from build123d import *

# Parameters (mm, degrees)
BASE_FLANGE1_DEPTH      = 2
EDGE_FLANGE1_DEPTH      = 40
EDGE_FLANGE1_BEND_DEPTH = 40
EDGE_FLANGE2_DEPTH      = 40
EDGE_FLANGE2_BEND_DEPTH = 40
SKETCH28_R              = 4
CUT_EXTRUDE1_DEPTH      = 2
SKETCH29_R              = 3
CUT_EXTRUDE2_DEPTH      = 2
SKETCH30_R              = 3
CUT_EXTRUDE3_DEPTH      = 2


# Sheet-metal steps are written as plain solids
with BuildPart() as part:
    # Sketch1 → Base-Flange1 (new body)
    with BuildSketch(Plane.XY):
        Polygon((-225, 173.125), (-225, -173.125), (-185, -173.125), (-185, -98.125), (185, -98.125), (185, -173.125), (225, -173.125), (225, 173.125), (185, 173.125), (185, 143.125), (-185, 143.125), (-185, 173.125), align=None)
    extrude(amount=-BASE_FLANGE1_DEPTH)

    # Edge-Flange1 section (across the edge) → Edge-Flange1 (add)
    with BuildSketch(Plane(origin=(-185, 173.339359354, 0), x_dir=(0, -0.49999999999999495, 0.8660254037844416), z_dir=(-1, 0, 0))):
        with BuildLine():
            Line((-2, 0.214359354), (-2, 38.954101615))
            Line((-2, 38.954101615), (0, 38.954101615))
            Line((0, 38.954101615), (0, 0.214359354))
            ThreePointArc((0, 0.214359354), (0.027259339, 0.007304118), (0.107179677, -0.185640646))
            Line((0.107179677, -0.185640646), (-1.624871131, -1.185640646))
            ThreePointArc((-1.624871131, -1.185640646), (-1.904592314, -0.510333972), (-2, 0.214359354))
        make_face()
    extrude(amount=EDGE_FLANGE1_DEPTH)

    # Edge-Flange1 section 2 (across the edge) → Edge-Flange1 bend (add)
    with BuildSketch(Plane(origin=(225, 173.339359354, 0), x_dir=(0, -0.49999999999999495, 0.8660254037844416), z_dir=(-1, 0, 0))):
        with BuildLine():
            Line((-2, 0.214359354), (-2, 38.954101615))
            Line((-2, 38.954101615), (0, 38.954101615))
            Line((0, 38.954101615), (0, 0.214359354))
            ThreePointArc((0, 0.214359354), (0.027259339, 0.007304118), (0.107179677, -0.185640646))
            Line((0.107179677, -0.185640646), (-1.624871131, -1.185640646))
            ThreePointArc((-1.624871131, -1.185640646), (-1.904592314, -0.510333972), (-2, 0.214359354))
        make_face()
    extrude(amount=EDGE_FLANGE1_BEND_DEPTH)

    # Edge-Flange2 section (across the edge) → Edge-Flange2 (add)
    with BuildSketch(Plane(origin=(-185, -173.339359354, -2), x_dir=(0, 0.49999999999999495, -0.8660254037844416), z_dir=(-1, 0, 0))):
        with BuildLine():
            Line((-2, 0.214359354), (-2, 29.464101615))
            Line((-2, 29.464101615), (0, 29.464101615))
            Line((0, 29.464101615), (0, 0.214359354))
            ThreePointArc((0, 0.214359354), (0.027259339, 0.007304118), (0.107179677, -0.185640646))
            Line((0.107179677, -0.185640646), (-1.624871131, -1.185640646))
            ThreePointArc((-1.624871131, -1.185640646), (-1.904592314, -0.510333972), (-2, 0.214359354))
        make_face()
    extrude(amount=EDGE_FLANGE2_DEPTH)

    # Edge-Flange2 section 2 (across the edge) → Edge-Flange2 bend (add)
    with BuildSketch(Plane(origin=(225, -173.339359354, -2), x_dir=(-1.3877787807814315e-15, 0.49999999999999495, -0.8660254037844416), z_dir=(-1, 0, 0))):
        with BuildLine():
            Line((-2, 0.214359354), (-2, 29.464101615))
            Line((-2, 29.464101615), (0, 29.464101615))
            Line((0, 29.464101615), (0, 0.214359354))
            ThreePointArc((0, 0.214359354), (0.027259339, 0.007304118), (0.107179677, -0.185640646))
            Line((0.107179677, -0.185640646), (-1.624871131, -1.185640646))
            ThreePointArc((-1.624871131, -1.185640646), (-1.904592314, -0.510333972), (-2, 0.214359354))
        make_face()
    extrude(amount=EDGE_FLANGE2_BEND_DEPTH)

    # Sketch28 → Cut-Extrude1 (cut)
    with BuildSketch(Plane.XY):
        with Locations((-205, 143.125)):
            Circle(SKETCH28_R)
        with Locations((-205, 110.125)):
            Circle(SKETCH28_R)
        with Locations((-205, 77.125)):
            Circle(SKETCH28_R)
        with Locations((-205, 44.125)):
            Circle(SKETCH28_R)
        with Locations((-205, 11.125)):
            Circle(SKETCH28_R)
        with Locations((-205, -21.875)):
            Circle(SKETCH28_R)
        with Locations((-205, -54.875)):
            Circle(SKETCH28_R)
        with Locations((-205, -87.875)):
            Circle(SKETCH28_R)
        with Locations((-205, -120.875)):
            Circle(SKETCH28_R)
        with Locations((-205, -153.875)):
            Circle(SKETCH28_R)
        with Locations(Location((205, -153.875, 0), (0, 0, 180))):
            Circle(SKETCH28_R)
        with Locations(Location((205, -120.875, 0), (0, 0, 180))):
            Circle(SKETCH28_R)
        with Locations(Location((205, -87.875, 0), (0, 0, 180))):
            Circle(SKETCH28_R)
        with Locations(Location((205, -54.875, 0), (0, 0, 180))):
            Circle(SKETCH28_R)
        with Locations(Location((205, -21.875, 0), (0, 0, 180))):
            Circle(SKETCH28_R)
        with Locations(Location((205, 11.125, 0), (0, 0, 180))):
            Circle(SKETCH28_R)
        with Locations(Location((205, 44.125, 0), (0, 0, 180))):
            Circle(SKETCH28_R)
        with Locations(Location((205, 77.125, 0), (0, 0, 180))):
            Circle(SKETCH28_R)
        with Locations(Location((205, 110.125, 0), (0, 0, 180))):
            Circle(SKETCH28_R)
        with Locations(Location((205, 143.125, 0), (0, 0, 180))):
            Circle(SKETCH28_R)
    extrude(amount=-CUT_EXTRUDE1_DEPTH, mode=Mode.SUBTRACT)

    # Sketch29 → Cut-Extrude2 (cut)
    with BuildSketch(Plane(origin=(0, -43.468814435, 75.290195146), x_dir=(1, 0, 0), z_dir=(0, -0.49999999999999517, 0.8660254037844416))):
        with Locations(Location((-215, -158.955519161, 0), (0, 0, 270))):
            Circle(SKETCH29_R)
        with Locations(Location((-215, -172.955519161, 0), (0, 0, 270))):
            Circle(SKETCH29_R)
        with Locations(Location((-195, -172.955519161, 0), (0, 0, 90))):
            Circle(SKETCH29_R)
        with Locations(Location((-195, -158.955519161, 0), (0, 0, 90))):
            Circle(SKETCH29_R)
        with Locations(Location((195, -172.955519161, 0), (0, 0, 270))):
            Circle(SKETCH29_R)
        with Locations(Location((195, -158.955519161, 0), (0, 0, 270))):
            Circle(SKETCH29_R)
        with Locations(Location((215, -158.955519161, 0), (0, 0, 90))):
            Circle(SKETCH29_R)
        with Locations(Location((215, -172.955519161, 0), (0, 0, 90))):
            Circle(SKETCH29_R)
    extrude(amount=-CUT_EXTRUDE2_DEPTH, mode=Mode.SUBTRACT)

    # Sketch30 → Cut-Extrude3 (cut)
    with BuildSketch(Plane(origin=(0, 44.334839838, -76.790195146), x_dir=(-1, 0, 0), z_dir=(0, 0.499999999999995, -0.8660254037844416))):
        with Locations(Location((-215, 176.700519161, 0), (0, 0, 90))):
            Circle(SKETCH30_R)
        with Locations(Location((-215, 162.700519161, 0), (0, 0, 90))):
            Circle(SKETCH30_R)
        with Locations(Location((-195, 162.700519161, 0), (0, 0, 270))):
            Circle(SKETCH30_R)
        with Locations(Location((-195, 176.700519161, 0), (0, 0, 270))):
            Circle(SKETCH30_R)
        with Locations(Location((195, 162.700519161, 0), (0, 0, 90))):
            Circle(SKETCH30_R)
        with Locations(Location((195, 176.700519161, 0), (0, 0, 90))):
            Circle(SKETCH30_R)
        with Locations(Location((215, 176.700519161, 0), (0, 0, 270))):
            Circle(SKETCH30_R)
        with Locations(Location((215, 162.700519161, 0), (0, 0, 270))):
            Circle(SKETCH30_R)
    extrude(amount=-CUT_EXTRUDE3_DEPTH, mode=Mode.SUBTRACT)


solid = part.part
Could you check a few things on this model? Use its own coordinates, in mm. A direction names the side the tool comes from. Give positions to 0.01 mm unless a question says otherwise; leave off trailing zeros. Order: outer loops, then holes, each group sorted by start corner. A loop starts at its lowest first (then second) coordinate and runs counter-clockwise, first axis right, second up.
1. Suppose I cut it at B-B (y = -69.5). List the corners of the cut face in (x, z) for me, plus the area to 3 significant figures.
2. Suppose I cut it at A-A (x = 10). List the corners of the cut face in (y, z) for me (3 decimals).
3. For faces 4 (the flat face through (-3, 2, 0)), 5 (the flat face through (185, 177, 1)), 6 (the flat face through (-3, 2, -2)), 7 (the flat face through (-185, -148.6, -1.6)), which set-ups out of +Z, -Z, +X, -X, +Y, -Y let a thin tool reach every point of the face, with its end or its side?
4. I need wall thicknesses on L1, parallel to Z at x = -200, y = -92. Which ranges of the line are inside material? Lowest first, please.
5. Will these pins go through, and if not, where does the flat tip stop? P1, Ø13, axis at x = 205, y = -21.875, coming from the -Z side; P2, Ø1.6, axis at x = 5, z = -0.5, coming from the -Y side (3 decimals); P3, Ø10.5, axis at x = 205, y = -87.875, coming from the +Z side.
6. We'd pull the mould along X, two halves only. Please class faces 1 (the flat face through (-204.72, -186.368, -9.522)), 2 (the flat face through (185, -148.6, -1.6)), 3 (the flat face through (-185, 177, 1)): pulls with the +X half, pulls with the -X half, needs draft (parallel to the pull), parting line crosses it, or undercut.
Solved:
1. outline: (-225, -2) - (225, -2) - (225, 0) - (-225, 0) - close
1. area: 900 mm2
2. outline: (-98.125, -2) - (143.125, -2) - (143.125, 0) - (-98.125, 0) - close
3. face 4: +Z, +X, -X, -Y
3. face 5: +Z, -Z, +Y
3. face 6: -Z, +X, -X, +Y
3. face 7: +Z, -Z, -Y
4. L1: z = -2 to 0
5. P1: stops at z = -2
5. P2: stops at y = -98.125
5. P3: stops at z = 0
6. face 1: needs draft
6. face 2: undercut
6. face 3: undercut
